from build123d import *

# Parameters (mm, degrees)
SKETCH1_W         = 5
SKETCH1_H         = 10.5
IDCHAMFER_SIZE    = 1.2
IDCHAMFERFAR_SIZE = 1.2


with BuildPart() as part:
    # Sketch1 → Base-Revolve (revolve)
    with BuildSketch(Plane.XY, mode=Mode.PRIVATE) as base_revolve_sk:
        with Locations((-2.5, 23.75)):
            Rectangle(SKETCH1_W, SKETCH1_H)
    revolve(base_revolve_sk.sketch.rotate(Axis((-34.925, 0, 0), (1, 0, 0)), 90), axis=Axis((-34.925, 0, 0), (1, 0, 0)))

    # IDChamfer
    idchamfer_edges = [part.edges().sort_by_distance(p)[0] for p in [
        (0, 0, -18.5),
    ]]
    chamfer(idchamfer_edges, length=IDCHAMFER_SIZE)

    # IDChamferFar
    idchamferfar_edges = [part.edges().sort_by_distance(p)[0] for p in [
        (-5, 0, -18.5),
    ]]
    chamfer(idchamferfar_edges, length=IDCHAMFERFAR_SIZE)


solid = part.part
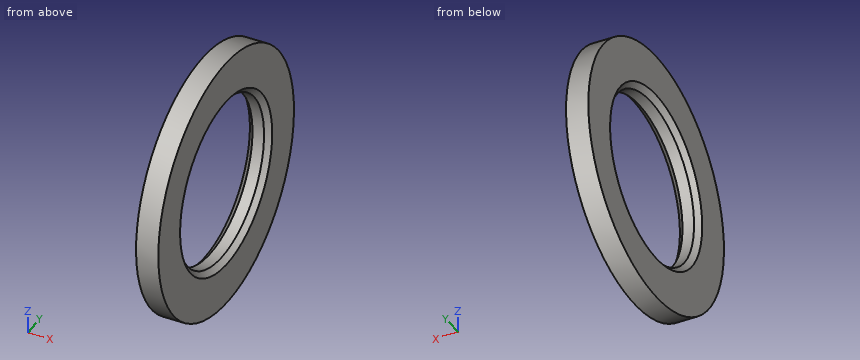
The listing builds one solid part. Answer for the finished solid, in the listing's coordinates (mm). Coordinates: 2 decimals unless noted, no trailing zeros. Loops run counter-clockwise (first coordinate to the right, second up) from the corner with the lowest first, then second, coordinate; pieces in that order, holes last. Notation, with made-up numbers: M -3,31.25 L 7,31.25 A32 cw 7,59.25 Z; hole C 12.5,-13.75 d4. An arc over 180 degrees is marked long. Answer in a Markdown table with one row per item.
1) Find section D-D (z = -25). Determine the outline of the cut face in (x, y).
Answers below:
| item | result |
|---|---|
| outline | M -5,-14.7 L 0,-14.7 L 0,14.7 L -5,14.7 Z |
2) Find section A-A (z = 0). Determine the outline of the cut face in (x, y), then the cut area to 3 significant figures.
Answers below:
| item | result |
|---|---|
| outline | M -5,-29 L 0,-29 L 0,-19.7 L -1.2,-18.5 L -3.8,-18.5 L -5,-19.7 Z; M -5,19.7 L -3.8,18.5 L -1.2,18.5 L 0,19.7 L 0,29 L -5,29 Z |
| area | 102 mm^2 |
3) Given pin 1 (1 mm diameter, centred on x = -4, z = -13.5, fed in from +Y); pin 2 (3 mm diameter, centred on x = -4.5, y = -20, fed in from +Z); pin 3 (1 mm diameter, centred on x = -1.5, z = -5.5, fed in from +Y), each flat-ended and moving along its own axis, determine where each tip first touches the part or whether it passes through.
Answers below:
| item | result |
|---|---|
| pin 1 | y = 25.92 |
| pin 2 | z = 22.33 |
| pin 3 | y = 28.57 |
4) Find the intervals of material crossed by probe 1 along Y at (x, z) = (-2.1, 0); probe 2 along Z at (x, y) = (-1.3, -7.5); probe 3 along Z at (x, y) = (-4.25, -7.5), in increasing order.
Answers below:
| item | result |
|---|---|
| probe 1 | -29 to -18.5, 18.5 to 29 |
| probe 2 | -28.01 to -16.91, 16.91 to 28.01 |
| probe 3 | -28.01 to -17.4, 17.4 to 28.01 |
5) Find section C-C (x = -2.45). Determine the outline of the cut face in (y, z).
Answers below:
| item | result |
|---|---|
| outline | C 0,0 d58; hole C 0,0 d37 |
